Part model, mm, in its own coordinate system. A direction names the side the tool comes from. Coordinates: 2 decimals unless noted, no trailing zeros. Order: outer loops, then holes, each group sorted by start corner. A loop starts at its lowest first (then second) coordinate and runs counter-clockwise, first axis right, second up.
from build123d import *

# Parameters (mm, degrees)
BOSS_EXTRUDE1_DEPTH = 72
SKETCH2_W           = 36
SKETCH2_H           = 36
BOSS_EXTRUDE3_DEPTH = 80
SKETCH4_R           = 9
CUT_EXTRUDE2_DEPTH  = 80
CUT_EXTRUDE3_DEPTH  = 80
RIB1_REACH          = 155.827
SKETCH7_WALL_W      = 405.799744174
SKETCH7_WALL_H      = 10
RIB4_REACH          = 155.827
SKETCH8_WALL_W      = 379.051427732
SKETCH8_WALL_H      = 10
RIB5_REACH          = 171.554
SKETCH12_WALL_W     = 379.578938684
SKETCH12_WALL_H     = 10


with BuildPart() as part:
    # Sketch1 → Boss-Extrude1 (new body)
    with BuildSketch(Plane.XY):
        with BuildLine():
            Line((-41.189710611, -1.813504823), (34.810289389, -1.813504823))
            Line((34.810289389, -1.813504823), (34.810289389, 8.186495177))
            Line((34.810289389, 8.186495177), (40.810289389, 8.186495177))
            ThreePointArc((40.810289389, 8.186495177), (58.810289389, 26.186495177), (76.810289389, 8.186495177))
            Line((76.810289389, 8.186495177), (112.810289389, 8.186495177))
            Line((112.810289389, 8.186495177), (112.810289389, 18.186495177))
            Line((112.810289389, 18.186495177), (80.627713618, 18.186495177))
            ThreePointArc((80.627713618, 18.186495177), (58.810289389, 32.186495177), (36.99286516, 18.186495177))
            Line((36.99286516, 18.186495177), (-41.189710611, 18.186495177))
            Line((-41.189710611, 18.186495177), (-41.189710611, -1.813504823))
        make_face()
    extrude(amount=-BOSS_EXTRUDE1_DEPTH)

    # Sketch2 → Boss-Extrude3 (add)
    with BuildSketch(Plane(origin=(0, 18.186495177, 0), x_dir=(1, 0, 0), z_dir=(0, 1, 0))):
        with Locations((-5.189710611, 36)):
            Rectangle(SKETCH2_W, SKETCH2_H)
    extrude(amount=BOSS_EXTRUDE3_DEPTH)

    # Sketch4 → Cut-Extrude2 (cut)
    with BuildSketch(Plane.XY.offset(-18)):
        with Locations((-5.189710611, 80.186495177)):
            Circle(SKETCH4_R)
    extrude(amount=-CUT_EXTRUDE2_DEPTH, mode=Mode.SUBTRACT)

    # Sketch5 → Cut-Extrude3 (cut)
    with BuildSketch(Plane.XY.offset(-18)):
        with BuildLine():
            Line((-10.189710611, 18.186495177), (-10.189710611, 62.186495177))
            Line((-10.189710611, 62.186495177), (-10.189710611, 62.894878711))
            ThreePointArc((-10.189710611, 62.894878711), (-19.577205181, 69.36984135), (-23.189710611, 80.186495177))
            Line((-23.189710611, 80.186495177), (-23.189710611, 18.186495177))
            Line((-23.189710611, 18.186495177), (-10.189710611, 18.186495177))
        make_face()
        with BuildLine():
            Line((-0.189710611, 62.186495177), (-0.189710611, 18.186495177))
            Line((-0.189710611, 18.186495177), (12.810289389, 18.186495177))
            Line((12.810289389, 18.186495177), (12.810289389, 80.186495177))
            ThreePointArc((12.810289389, 80.186495177), (9.197783959, 69.36984135), (-0.189710611, 62.894878711))
            Line((-0.189710611, 62.894878711), (-0.189710611, 62.186495177))
        make_face()
        with BuildLine():
            Line((12.810289389, 98.186495177), (-5.1897106, 98.186495177))
            ThreePointArc((-5.1897106, 98.186495177), (7.538211454, 92.914417234), (12.810289389, 80.186495177))
            Line((12.810289389, 80.186495177), (12.810289389, 98.186495177))
        make_face()
        with BuildLine():
            Line((-23.189710611, 98.186495177), (-23.189710611, 80.186495177))
            ThreePointArc((-23.189710611, 80.186495177), (-17.917632668, 92.914417242), (-5.1897106, 98.186495177))
            Line((-5.1897106, 98.186495177), (-23.189710611, 98.186495177))
        make_face()
    extrude(amount=-CUT_EXTRUDE3_DEPTH, mode=Mode.SUBTRACT)

    # Sketch7 wall → Rib1 (add, up to next)
    with BuildSketch(Plane(origin=(41.606445938, 59.088634331, -36), x_dir=(0.709625674027, -0.704578883278, 0), z_dir=(0.704578883278, 0.709625674027, 0)), mode=Mode.PRIVATE) as rib1_sk1:
        Rectangle(SKETCH7_WALL_W, SKETCH7_WALL_H)
    rib1_tool1 = extrude(rib1_sk1.sketch, amount=-RIB1_REACH, mode=Mode.PRIVATE) - part.part
    add(rib1_tool1.solids().sort_by_distance((41.606445938, 59.088634331, -36))[0])

    # Sketch8 wall → Rib4 (add, up to next)
    with BuildSketch(Plane(origin=(-31.858144991, 51.606876429, -36), x_dir=(-0.268931250293, -0.963159375501, 0), z_dir=(0.963159375501, -0.268931250293, 0)), mode=Mode.PRIVATE) as rib4_sk1:
        Rectangle(SKETCH8_WALL_W, SKETCH8_WALL_H)
    rib4_tool1 = extrude(rib4_sk1.sketch, amount=RIB4_REACH, mode=Mode.PRIVATE) - part.part
    add(rib4_tool1.solids().sort_by_distance((-31.858144991, 51.606876429, -36))[0])

    # Sketch12 wall → Rib5 (add, up to next)
    with BuildSketch(Plane(origin=(-5.189710611, 35.186495177, -9), x_dir=(0, -0.883787916347, 0.467887720419), z_dir=(0, 0.467887720419, 0.883787916347)), mode=Mode.PRIVATE) as rib5_sk1:
        Rectangle(SKETCH12_WALL_W, SKETCH12_WALL_H)
    rib5_tool1 = extrude(rib5_sk1.sketch, amount=-RIB5_REACH, mode=Mode.PRIVATE) - part.part
    add(rib5_tool1.solids().sort_by_distance((-5.189710611, 35.186495177, -9))[0])


solid = part.part
Q1. Wall check: line 1 along X through (y, z) = (24, -12); line 2 along X through (y, z) = (23, -42); line 3 along Y through (x, z) = (-21, -2.5). Give the ranges that are in metal, low to high.
Results list:
line 1: x = -10.19 to -0.19, 40.76 to 50.21, 67.41 to 76.86
line 2: x = -10.19 to -0.19, 39.93 to 48.58, 69.04 to 77.69
line 3: y = -1.81 to 18.19
Q2. Cut at D-D on y = 21. Write the cut outline in (x, z), and give its area (3 significant figures).
Results list:
outline: (-40.4, -41) - (-10.19, -41) - (-10.19, -54) - (-0.19, -54) - (-0.19, -41) - (38.52, -41) - (38.52, -72) - (46.17, -72) - (46.17, 0) - (38.52, 0) - (38.52, -31) - (-0.19, -31) - (-0.19, -1.49) - (-10.19, -1.49) - (-10.19, -31) - (-40.4, -31) - close; (71.45, -72) - (79.1, -72) - (79.1, 0) - (71.45, 0) - close
area: 2,320 mm2
Q3. Which spindle directions (+Z, -Z, +X, -X, +Y, -Y) get a long thin tool onto all of the face, cutting with end or side? Do faces 4 (the face through (97, 18.186, -35)), 5 (the face through (-2, 18.186, -56)), 6 (the face through (-5, 67, -54)), 7 (the face through (95, 8.186, -35)), 8 (the face through (-10.19, 39, -19)). Say none if no direction does.
Results list:
face 4: +Z, -Z, +X, +Y
face 5: -Z
face 6: -Z, -X, +Y
face 7: +Z, -Z, +X, -Y
face 8: +Z, -X
Q4. Pin check, flat tips, straight feed: pin 1 Ø12 at (y, z) = (87, -37.5) entering from -X; pin 2 Ø25 at (x, y) = (-27, 59) entering from +Z; pin 3 Ø18 at (x, y) = (-7.5, 46) entering from -Z. Stop position of each tip, or through.
Results list:
pin 1: stops at x = -23.65
pin 2: stops at z = -18
pin 3: stops at z = -54
Q5. Cut at B-B on y = 82.5. Write the cut outline in (x, z).
Results list:
outline: (-23.23, -41) - (-23.04, -41) - (-23.04, -54) - (-13.89, -54) - (-13.89, -18) - (-23.04, -18) - (-23.04, -31) - (-23.23, -31) - close; (3.51, -54) - (12.66, -54) - (12.66, -41) - (18.03, -41) - (18.03, -31) - (12.66, -31) - (12.66, -18) - (3.51, -18) - close
Q6. Cut at A-A on z = -51.5. Write the cut outline in (x, y), and give its area (3 significant figures).
Results list:
outline: (-41.19, -1.81) - (34.81, -1.81) - (34.81, 8.19) - (40.81, 8.19) arc R18 cw to (76.81, 8.19) - (112.81, 8.19) - (112.81, 18.19) - (80.63, 18.19) arc R24 ccw to (36.99, 18.19) - (-0.19, 18.19) - (-0.19, 62.89) arc R18 ccw (long way) to (-10.19, 62.89) - (-10.19, 18.19) - (-41.19, 18.19) - close; hole circle Ø18 at (-5.19, 80.19)
area: 3,440 mm2
Q7. Mould opens along Y. For faces 1 (the face through (-6.36, 89.11, -35.75)), 2 (the face through (-5.12, 35.424, -9.126)), 3 (the face through (-4, -1.814, -35)) say: pulls with the +Y half, pulls with the -Y half, needs draft (parallel to the pull), parting line crosses it, or undercut.
Results list:
face 1: undercut
face 2: pulls with the +Y half
face 3: pulls with the -Y half
Q8. Cut at C-C on x = -18. Write the cut outline in (y, z).
Results list:
outline: (-1.81, -72) - (18.19, -72) - (18.19, -41) - (67.54, -41) - (67.54, -54) - (92.83, -54) - (92.83, -18) - (67.54, -18) - (67.54, -31) - (18.19, -31) - (18.19, 0) - (-1.81, 0) - close
